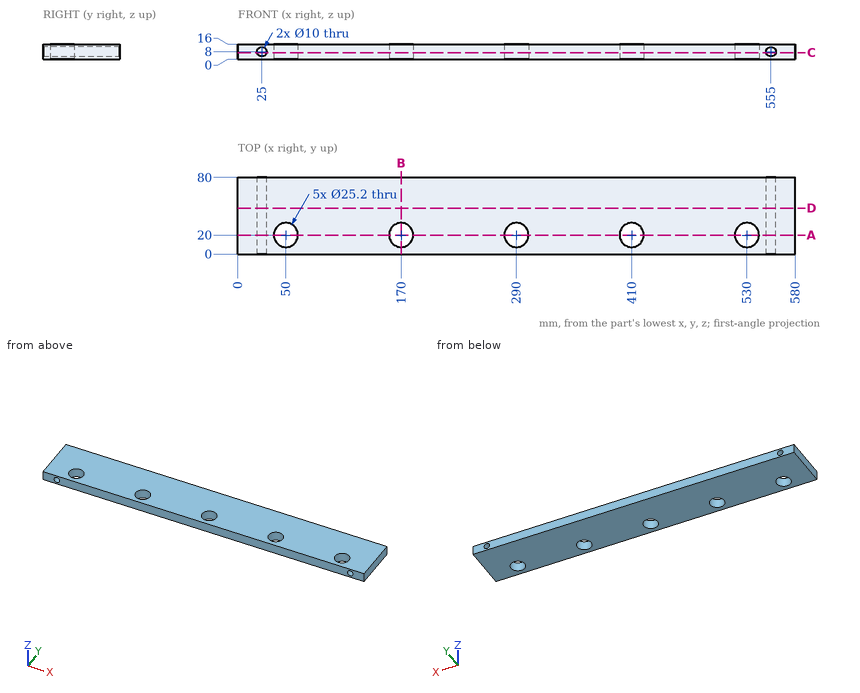
Here's the drawing with two shaded views (mm, measured from the low corner). I have some questions. Coordinates: 2 decimals unless noted, no trailing zeros. Write each loop counter-clockwise with the first axis right and the second up, starting at its lowest first coordinate (ties: lowest second). Pieces come first, ordered by that corner, then holes. Notation, with made-up numbers: (34.5, -14.5) -> (86.5, -14.5) arc R14 ccw to (86.5, -4.5) -> close; hole circle Ø5 at (-21, 70.5). An arc over 180 degrees is marked (long way). Write item = value, one per line. Start each with the question number.
(1) I want a section at C-C (z = 7). Please give me the cut outline in (x, y), plus the area to 3 significant figures.
(2) I want a section at D-D (y = 48). Please give me the cut outline in (x, z).
(3) I want a section at B-B (x = 170). Please give me the cut outline in (y, z), plus the area to 3 significant figures.
(4) I want a section at A-A (y = 20). Please give me the cut outline in (x, z).
(5) I need wall thicknesses on line 1 (X direction, y = 55.5, z = 8); line 2 (Z direction, x = 25, y = 59); line 3 (X direction, y = 59, z = 10.75). Which ranges of each line are inside material? Lowest first, please. Write a range as [from, to].
Result set:
q1.outline = (0, 0) -> (20.1, 0) -> (20.1, 80) -> (0, 80) -> close; (29.9, 0) -> (550.1, 0) -> (550.1, 80) -> (29.9, 80) -> close; (559.9, 0) -> (580, 0) -> (580, 80) -> (559.9, 80) -> close; hole circle Ø25.2 at (50, 20); hole circle Ø25.2 at (170, 20); hole circle Ø25.2 at (290, 20); hole circle Ø25.2 at (410, 20); hole circle Ø25.2 at (530, 20)
q1.area = 42,300 mm2
q2.outline = (0, 0) -> (580, 0) -> (580, 16) -> (0, 16) -> close; hole circle Ø10 at (25, 8); hole circle Ø10 at (555, 8)
q3.outline = (0, 0) -> (7.4, 0) -> (7.4, 16) -> (0, 16) -> close; (32.6, 0) -> (80, 0) -> (80, 16) -> (32.6, 16) -> close
q3.area = 877 mm2
q4.outline = (0, 0) -> (37.4, 0) -> (37.4, 16) -> (0, 16) -> close; (62.6, 0) -> (157.4, 0) -> (157.4, 16) -> (62.6, 16) -> close; (182.6, 0) -> (277.4, 0) -> (277.4, 16) -> (182.6, 16) -> close; (302.6, 0) -> (397.4, 0) -> (397.4, 16) -> (302.6, 16) -> close; (422.6, 0) -> (517.4, 0) -> (517.4, 16) -> (422.6, 16) -> close; (542.6, 0) -> (580, 0) -> (580, 16) -> (542.6, 16) -> close; hole circle Ø10 at (25, 8); hole circle Ø10 at (555, 8)
q5.line_1 = [0, 20], [30, 550], [560, 580]
q5.line_2 = [0, 3], [13, 16]
q5.line_3 = [0, 20.82], [29.18, 550.82], [559.18, 580]
